from build123d import *

# Parameters (mm, degrees)
SKETCH1_R               = 9
BOSS_EXTRUDE1_DEPTH     = 12.5
SKETCH2_R               = 9
BOSS_EXTRUDE2_DEPTH     = 10
CUT_EXTRUDE1_DEPTH      = 26.850531909
CUT_EXTRUDE1_DEPTH_BACK = 26.850531909
SKETCH3_R               = 2


with BuildPart() as part:
    # Sketch1 → Boss-Extrude1 (new body)
    with BuildSketch(Plane.XY):
        Circle(SKETCH1_R)
    extrude(amount=BOSS_EXTRUDE1_DEPTH)

    # Sketch2 → Boss-Extrude2 (add)
    with BuildSketch(Plane.XY.offset(12.5)):
        Circle(SKETCH2_R)
    extrude(amount=BOSS_EXTRUDE2_DEPTH)

    # Sketch3 → Cut-Extrude1 (cut, two sides: drawn at the far end of the back side and taken through both)
    with BuildSketch(Plane(origin=(0, 0, 0), x_dir=(1, 0, 0), z_dir=(0, 1, 0)).offset(-CUT_EXTRUDE1_DEPTH_BACK)):
        with Locations(Location((0, -17.5, 0), (0, 0, 270))):
            Circle(SKETCH3_R)
    extrude(amount=CUT_EXTRUDE1_DEPTH + CUT_EXTRUDE1_DEPTH_BACK, mode=Mode.SUBTRACT)

    # Mirror1: part across plane


with BuildPart() as part_1:
    add(part.part)
    add(part.part.mirror(Plane.XY))


solid = part_1.part
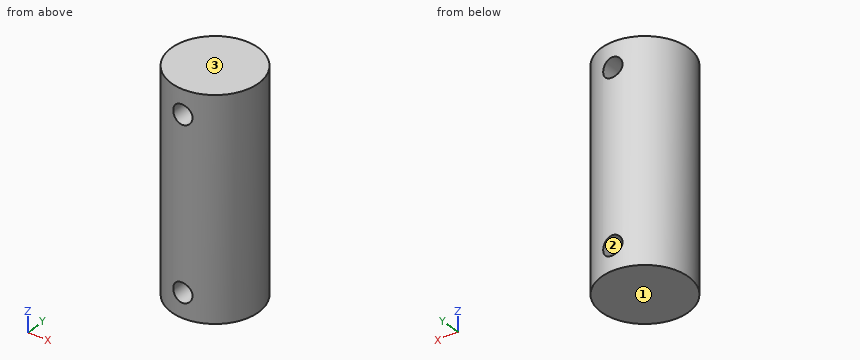
The listing builds one solid part. Answer for the finished solid, in the listing's coordinates (mm). Face numbers are marked on the shaded views. Round coordinates to 2 decimals unless told otherwise and drop trailing zeros. Order: outer loops, then holes, each group sorted by start corner. A loop starts at its lowest first (then second) coordinate and runs counter-clockwise, first axis right, second up. Notation, with made-up numbers: (25.5, -19.5) -> (41.5, -19.5) arc R22 ccw to (41.5, -2.5) -> close; hole circle Ø3 at (83, 75.25). An arc over 180 degrees is marked (long way). Write each question's results on one line, items separated by ' | '. Start each with the question number.
Q1. Each of these flat-tipped pins is pushed along its axis until it touches: pin 1 (4 mm diameter, centred on y = 4.5, z = 2, fed in from -X); pin 2 (3 mm diameter, centred on y = -5, z = 13, fed in from +X); pin 3 (8 mm diameter, centred on x = 7, z = 1.5, fed in from -Y); pin 4 (8 mm diameter, centred on y = -3.5, z = 5, fed in from -X). Where does it stop, or does it pass through?
Q2. Find section C-C (z = -8). Determine the outline of the cut face in (x, y).
Q3. Straight lines are drawn through the part: probe 1 along Z at (x, y) = (0, 1.75); probe 2 along Z at (x, y) = (1.5, -0.5); probe 3 along X at (y, z) = (5, 17.5). For each, find the intervals that lie inside material, in ascending order. Write a range as from..to.
Q4. Find section B-B (y = 0). Determine the outline of the cut face in (x, z).
Q5. Find section A-A (x = 0). Determine the outline of the cut face in (y, z), then the cut area to 3 significant figures.
Q6. Find section D-D (x = -5.25). Determine the outline of the cut face in (y, z).
Q7. The mould has two halves that part along Z. Classify the marked faces 1, 2 and 3: pulls with the +Z half, pulls with the -Z half, needs draft (parallel to the pull), parting line crosses it, or undercut.
Worked answers:
1) pin 1: stops at x = -8.65 | pin 2: stops at x = 8.29 | pin 3: stops at y = -8.49 | pin 4: stops at x = -9
2) outline: circle Ø18 at (0, 0)
3) probe 1: z = -22.5..-19.5, -15.5..15.5, 19.5..22.5 | probe 2: z = -22.5..-18.82, -16.18..16.18, 18.82..22.5 | probe 3: x = -7.48..-2, 2..7.48
4) outline: (-9, -22.5) -> (9, -22.5) -> (9, 22.5) -> (-9, 22.5) -> close; hole circle Ø4 at (0, -17.5); hole circle Ø4 at (0, 17.5)
5) outline: (-9, -22.5) -> (9, -22.5) -> (9, -19.5) -> (-9, -19.5) -> close; (-9, -15.5) -> (9, -15.5) -> (9, 15.5) -> (-9, 15.5) -> close; (-9, 19.5) -> (9, 19.5) -> (9, 22.5) -> (-9, 22.5) -> close | area: 666 mm2
6) outline: (-7.31, -22.5) -> (7.31, -22.5) -> (7.31, 22.5) -> (-7.31, 22.5) -> close
7) face 1: pulls with the -Z half | face 2: undercut | face 3: pulls with the +Z half
